from build123d import *

# Parameters (mm, degrees)
SKETCH_R        = 5.130877
PAD_DEPTH       = 26
SKETCH002_R     = 1.142124
SKETCH003_R     = 8.361882
PAD001_DEPTH    = 40
PAD002_DEPTH    = 2
POCKET_DEPTH    = 10.5
SKETCH007_R     = 5.632133
POCKET001_DEPTH = 5


with BuildPart() as part:
    # Sketch → Pad (new body)
    with BuildSketch(Plane.XY):
        Circle(SKETCH_R)
    extrude(amount=PAD_DEPTH)

    # Sketch002 (on DatumPlane) → Groove (revolve, cut)
    with BuildSketch(Plane(origin=(0, 0, 13), x_dir=(1, 0, 0), z_dir=(0, -1, 0))):
        with Locations((5.337208, 0)):
            Circle(SKETCH002_R)
    revolve(axis=Axis((0, 0, 13), (0, 0, 1)), mode=Mode.SUBTRACT)

    # Sketch003 (on Face2 of Groove) → Pad001 (join)
    with BuildSketch(Plane(origin=(0, 0, 0), x_dir=(1, 0, 0), z_dir=(0, 0, -1))):
        Circle(SKETCH003_R)
    extrude(amount=PAD001_DEPTH)

    # Sketch004 (on DatumPlane) → Groove001 (revolve, cut)
    with BuildSketch(Plane(origin=(0, 0, 13), x_dir=(1, 0, 0), z_dir=(0, -1, 0))):
        Polygon((-2.098671, 66.083956), (-2.098671, -33.279097), (0, -36.189228), (0, -33.279097), (0, 66.139438), (0, 66.083956), align=None)
    revolve(axis=Axis((0, 0, 13), (0, 0, 1)), mode=Mode.SUBTRACT)

    # Sketch005 (on DatumPlane) → Pad002 (join, symmetric)
    with BuildSketch(Plane(origin=(0, 0, 13), x_dir=(1, 0, 0), z_dir=(0, -1, 0))):
        with BuildLine():
            Line((7.000219, -29.542121), (49.71245, -70.147492))
            ThreePointArc((50.443017, -85.924472), (68.024657, -77.204934), (49.71245, -70.147492))
            Line((7.000219, -52.373556), (50.443017, -85.924472))
            Line((7.000219, -29.542121), (7.000219, -52.373556))
        make_face()
    extrude(amount=PAD002_DEPTH, both=True)

    # Sketch006 (on DatumPlane) → Pocket (cut, symmetric)
    with BuildSketch(Plane(origin=(0, 0, 13), x_dir=(1, 0, 0), z_dir=(0, -1, 0))):
        Polygon((-10.626366, -38.553432), (62.605824, -94.891693), (-10.165777, -94.891693), align=None)
    extrude(amount=POCKET_DEPTH, both=True, mode=Mode.SUBTRACT)

    # Sketch007 (on Face3 of Pocket) → Pocket001 (cut)
    with BuildSketch(Plane(origin=(0, 2, 0), x_dir=(-1, 0, 0), z_dir=(0, 1, 0))):
        with Locations((-57.609379, -65.024849)):
            Circle(SKETCH007_R)
    extrude(amount=-POCKET001_DEPTH, mode=Mode.SUBTRACT)


solid = part.part
Source: CAD feature listing. Evaluate the final solid. Frame: model axes, mm. A direction names the side the tool comes from. Give positions to 0.01 mm unless a question says otherwise; leave off trailing zeros. Loops run counter-clockwise (first coordinate to the right, second up) from the corner with the lowest first, then second, coordinate; pieces in that order, holes last. Notation, with made-up numbers: (-39, 29) -> (-15, 29) arc R4 ccw to (-15, 36) -> close; hole circle Ø9 at (20.25, 40). An arc over 180 degrees is marked (long way). Use a Markdown table: item, result. Add a question column.
1) Reachability of faces 5 (the face through (-1.11, -5.01, 19.98)), 6 (the face through (67.9, 0, -63)), 7 (the face through (36, -2, -51)) from +Z, -Z, +X, -X, +Y, -Y: full face, straight path, thin tool, end or side. Return the list, or none.
2) Line query: line 1 along Y through (x, z) = (0, 8); line 2 along Y through (x, z) = (0, -7). Output: solid intervals per line, ascending. Write a range as [from, to].
3) Section query D-D, the plane y = -6.25. Return the cut outline in (x, z), then the cut area to 3 significant figures.
4) Section query A-A, the plane x = 59.5. Return the cut outline in (y, z).
5) Pull-direction query (Z, two-part tool) for faces 1 (the face through (36, 2, -51)), 2 (the face through (15.08, -0.12, -45.33)), 3 (the face through (0.123, 0.555, -22.401)), 4 (the face through (54.582, 0.028, -60.276)); classes: +Z half, -Z half, draft (parallel to the pull), parting line (faces both ways), or undercut.
6) Section query C-C, the plane x = 12. Return the cut outline in (y, z).
7) Section query B-B, the plane z = -29. Return the cut outline in (x, y).
8) First-contact query: pin 1 (1.5 mm diameter, centred on x = 20.5, y = 0.5, fed in from +Z); pin 2 (8 mm diameter, centred on y = -5, z = -60.5, fed in from -X); pin 3 (1.5 mm diameter, centred on y = 4, z = -51, fed in from +X); pin 4 (8 mm diameter, centred on x = 26, y = 5, fed in from +Z). Flat tips, straight axial feed; report the tip coordinate or a pass-through.
Numbers:
| question | item | result |
|---|---|---|
| 1 | face 5 | +Z |
| 1 | face 6 | +Y, -Y |
| 1 | face 7 | +Z, -Z, +X, -Y |
| 2 | line 1 | y = [-5.13, -2.1], [2.1, 5.13] |
| 2 | line 2 | y = [-8.36, -2.1], [2.1, 8.36] |
| 3 | outline | (-5.56, -29.45) -> (5.56, -38) -> (5.56, 0) -> (-5.56, 0) -> close |
| 3 | area | 375 mm2 |
| 4 | outline | (-2, -75.19) -> (2, -75.19) -> (2, -70.33) -> (-2, -70.33) -> close; (-2, -59.72) -> (2, -59.72) -> (2, -54.21) -> (-2, -54.21) -> close |
| 5 | face 1 | draft |
| 5 | face 2 | -Z half |
| 5 | face 3 | +Z half |
| 5 | face 4 | undercut |
| 6 | outline | (-2, -42.96) -> (2, -42.96) -> (2, -21.3) -> (-2, -21.3) -> close |
| 7 | outline | (-6.15, -5.67) arc R8.36 ccw to (8.12, -2) -> (20.1, -2) -> (20.1, 2) -> (8.12, 2) arc R8.36 ccw to (-6.15, 5.67) -> close |
| 8 | pin 1 | stops at z = -28.66 |
| 8 | pin 2 | stops at x = 31.36 |
| 8 | pin 3 | passes through |
| 8 | pin 4 | stops at z = -32.09 |
